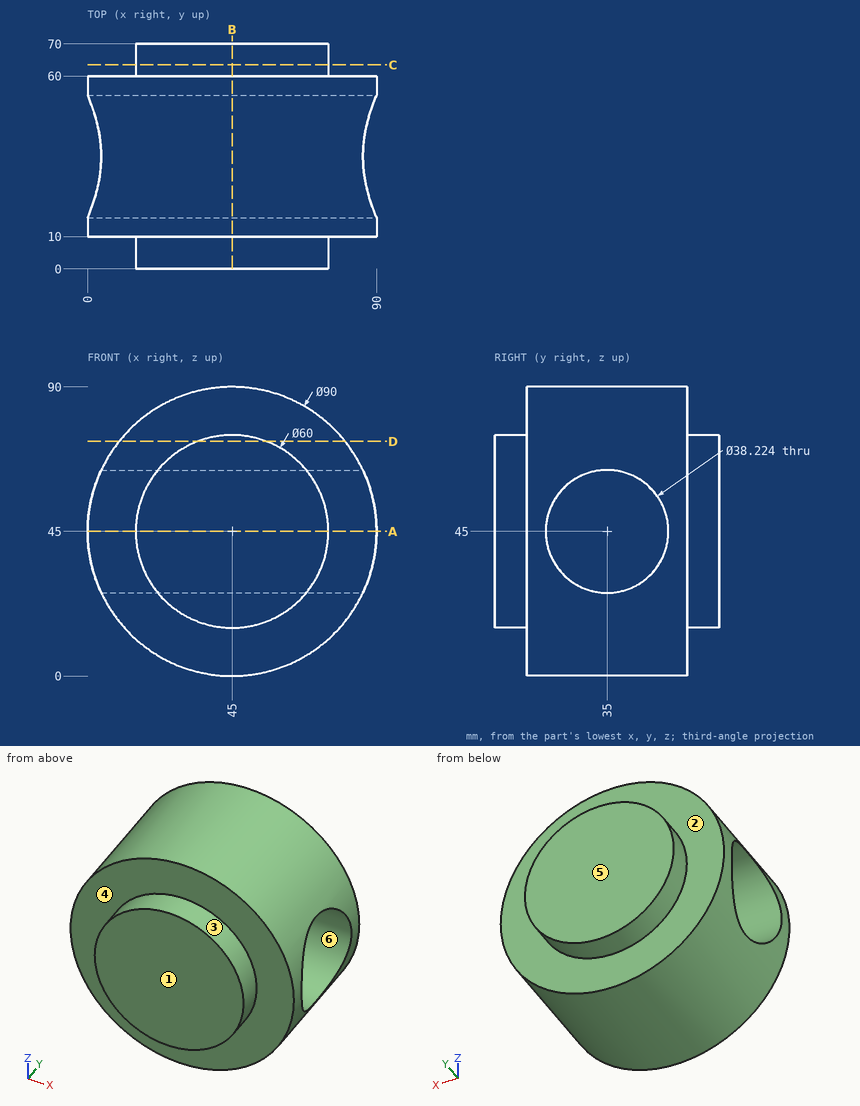
Job drawing, mm, ordinate dimensions from the low corner. One solid piece. A direction names the side the tool comes from. Give positions to 0.01 mm unless a question says otherwise; leave off trailing zeros. Order: outer loops, then holes, each group sorted by start corner. A loop starts at its lowest first (then second) coordinate and runs counter-clockwise, first axis right, second up. Notation, with made-up numbers: (60.5, 2.25) - (70.5, 2.25) arc R25 cw to (70.5, 20.25) - close; hole circle Ø4 at (-14, 46.5). An arc over 180 degrees is marked (long way). Answer in a Markdown table with one row per item.
1. Saw through at D-D, the plane z = 73. Give the cut face in (x, y), plus the area to 3 significant figures.
Data:
| item | result |
|---|---|
| outline | (9.77, 10) - (34.23, 10) - (34.23, 0) - (55.77, 0) - (55.77, 10) - (80.23, 10) - (80.23, 60) - (55.77, 60) - (55.77, 70) - (34.23, 70) - (34.23, 60) - (9.77, 60) - close |
| area | 3,950 mm² |
2. Saw through at A-A, the plane z = 45. Give the cut face in (x, y), plus the area to 3 significant figures.
Data:
| item | result |
|---|---|
| outline | (0, 10) - (15, 10) - (15, 0) - (75, 0) - (75, 10) - (90, 10) - (90, 15.89) - (0, 15.89) - close; (0, 54.11) - (90, 54.11) - (90, 60) - (75, 60) - (75, 70) - (15, 70) - (15, 60) - (0, 60) - close |
| area | 2,260 mm² |
3. Pull direction Y, two halves, no side cores. Call the marked faces 3, 4, 5 and 6: pulls with the +Y half, pulls with the -Y half, needs draft (parallel to the pull), parting line crosses it, or undercut.
Data:
| item | result |
|---|---|
| face 3 | needs draft |
| face 4 | pulls with the -Y half |
| face 5 | pulls with the +Y half |
| face 6 | undercut |
4. Probe probe 1 along Z at (x, y) = (28, 35) (1 decimal); probe 2 along Z at (x, y) = (68, 32.5); probe 3 along Y at (x, z) = (81, 47.5). List the from-to ranges inside material, lowest first. Write a range as [from, to].
Data:
| item | result |
|---|---|
| probe 1 | z = [3.3, 25.9], [64.1, 86.7] |
| probe 2 | z = [6.32, 26.05], [63.95, 83.68] |
| probe 3 | y = [10, 16.05], [53.95, 60] |
5. Tool access for the marked faces 1 and 2: list every direction of +Z, -Z, +X, -X, +Y, -Y with a clear straight run to the whole face (end or side of a thin tool).
Data:
| item | result |
|---|---|
| face 1 | +Z, -Z, +X, -X, -Y |
| face 2 | +Y |
6. Saw through at B-B, the plane x = 45. Give the cut face in (y, z), plus the area to 3 significant figures.
Data:
| item | result |
|---|---|
| outline | (0, 15) - (10, 15) - (10, 0) - (60, 0) - (60, 15) - (70, 15) - (70, 75) - (60, 75) - (60, 90) - (10, 90) - (10, 75) - (0, 75) - close; hole circle Ø38.22 at (35, 45) |
| area | 4,550 mm² |
7. Flat gauge pins, fed straight in: pin 1 (6 mm diameter, centred on y = 55.5, z = 53.5, fed in from -X); pin 2 (1.5 mm diameter, centred on x = 42, y = 10.5, fed in from +Z); pin 3 (5 mm diameter, centred on x = 38, y = 40, fed in from +Z). Where does each tip first touch, or does it go through?
Data:
| item | result |
|---|---|
| pin 1 | stops at x = 0.34 |
| pin 2 | stops at z = 89.94 |
| pin 3 | stops at z = 89.77 |
8. Saw through at C-C, the plane y = 63.5. Give the cut face in (x, z), plus the area to 3 significant figures.
Data:
| item | result |
|---|---|
| outline | circle Ø60 at (45, 45) |
| area | 2,830 mm² |
